Work out the finished part from the listing and answer in its coordinate system (mm). A direction names the side the tool comes from. Give positions to 0.01 mm unless a question says otherwise; leave off trailing zeros. Loops run counter-clockwise (first coordinate to the right, second up) from the corner with the lowest first, then second, coordinate; pieces in that order, holes last. Notation, with made-up numbers: M 84,9 L 113,9 A7 ccw 113,16 Z; hole C -32.5,87 d5. An arc over 180 degrees is marked long. Write item = value, one per line. Start each with the question number.
1. Consider L1, parallel to Z at x = 93, y = -0.75; L2, parallel to X at y = 3, z = -29; L3, parallel to Z at x = 218, y = 1. Determine where each line is inside the solid, lowest interval first. Write a range as [from, to].
2. Flat-ended cylindrical pins translate along their axes: pin 1 Ø5 at (y, z) = (-2, -31.5) entering from -X; pin 2 Ø3 at (x, y) = (196, -2.5) entering from +Z; pin 3 Ø5 at (y, z) = (0, -29.5) entering from +X. Find the tip coordinate at first contact, or state that the pin passes through.
3. For faces 1 (the face through (240, 0, -60)), 2 (the face through (115, 0, -30)), 3 (the face through (191, 0, -55)), determine the directions among +Z, -Z, +X, -X, +Y, -Y from which every point of the face is accessible in a straight line to the end or side of a thin tool.
4. Section C-C on z = -32.5 is taken. Determine the outline of the cut face in (x, y), plus the area to 3 significant figures.
5. Section B-B on x = 204.5 is taken. Determine the outline of the cut face in (y, z).
6. Section A-A on y = -0.5 is taken. Determine the outline of the cut face in (x, z).
```python
from build123d import *

# Parameters (mm, degrees)
SKETCH3_W = 10
SKETCH3_H = 10


with BuildPart() as part:
    # Sweep3: sweep along a path in Sketch1
    with BuildLine(Plane(origin=(0, 0, 0), x_dir=(1, 0, 0), z_dir=(0, 1, 0))) as sweep3_path:
        Line((0, 0), (100, 0))
        ThreePointArc((100, 0), (114.142135624, 5.857864376), (120, 20))
        Line((120, 20), (120, 40))
        ThreePointArc((120, 40), (125.857864376, 54.142135624), (140, 60))
        Line((140, 60), (240, 60))
    # Sketch3 → Sweep3 (sweep)
    with BuildSketch(Plane(origin=(0, 0, 0), x_dir=(0, 0, -1), z_dir=(1, 0, 0))):
        Rectangle(SKETCH3_W, SKETCH3_H)
    sweep(path=sweep3_path.line)


solid = part.part
```
Verdict:
q1.L1 = [-5, 5]
q1.L2 = [115, 125]
q1.L3 = [-65, -55]
q2.pin_1 = 115
q2.pin_2 = -55
q2.pin_3 = 125
q3.face_1 = +Z, -Z, +X, +Y, -Y
q3.face_2 = -Z, -X, +Y, -Y
q3.face_3 = +Z, +X, +Y, -Y
q4.outline = M 115,-5 L 125,-5 L 125,5 L 115,5 Z
q4.area = 100 mm2
q5.outline = M -5,-65 L 5,-65 L 5,-55 L -5,-55 Z
q6.outline = M 0,-5 L 100,-5 A15 cw 115,-20 L 115,-40 A25 ccw 140,-65 L 240,-65 L 240,-55 L 140,-55 A15 cw 125,-40 L 125,-20 A25 ccw 100,5 L 0,5 Z
